from build123d import *

# Parameters (mm, degrees)
BOSS_EXTRUDE1_DEPTH = 6.35
FILLET1_R           = 3.81


with BuildPart() as part:
    # Sketch3 → Boss-Extrude1 (new body)
    with BuildSketch(Plane(origin=(809.076030053, 943.560396052, 1278.390464274), x_dir=(-1, 0, 0), z_dir=(0, 0.4075747752498649, -0.913171836282757))):
        with BuildLine():
            Line((137.874265639, -126.392405854), (-26.505638525, -18.937567822))
            Line((-26.505638525, -18.937567822), (-39.07644953, -10.720052017))
            ThreePointArc((-39.07644953, -10.720052017), (-20.260111199, -2.728624711), (0, 0))
            Line((0, 0), (320.198396744, 0))
            ThreePointArc((320.198396744, 0), (340.458416927, -2.728663039), (359.274618149, -10.720195518))
            Line((359.274618149, -10.720195518), (346.703910708, -18.937649247))
            Line((346.703910708, -18.937649247), (182.324265639, -126.392391447))
            ThreePointArc((182.324265639, -126.392391447), (160.099261742, -114.368537545), (137.874265639, -126.392405854))
        make_face()
    extrude(amount=BOSS_EXTRUDE1_DEPTH)

    # Fillet1
    fillet1_edges = [part.edges().sort_by_distance(p)[0] for p in [
        (671.201764414, 829.436460617, 1223.976787284),
        (848.152479583, 935.065196378, 1271.121920902),
        (449.801411904, 935.065065337, 1271.121862415),
        (626.751764414, 829.436473773, 1223.976793156),
    ]]
    fillet(fillet1_edges, radius=FILLET1_R)


solid = part.part
Read the model definition and answer for the solid it produces. Units are mm, in the model's axes. Round coordinates to 2 decimals unless told otherwise and drop trailing zeros. Write each loop counter-clockwise with the first axis right and the second up, starting at its lowest first coordinate (ties: lowest second). Pieces come first, ordered by that corner, then holes. Notation, with made-up numbers: M -36.75,43 L 2.25,43 A9 cw 2.25,52 Z; hole C -36,21.25 d8. An arc over 180 degrees is marked long. Use a Markdown table: item, result.
1) Flat-ended cylindrical pins translate along their axes: pin 1 (2 mm diameter, centred on x = 664, y = 861.5, fed in from -Z); pin 2 (5 mm diameter, centred on x = 625, y = 925, fed in from -Z); pin 3 (10 mm diameter, centred on x = 688.5, z = 1254.5, fed in from +Y). Find the tip coordinate at first contact, or state that the pin passes through.
Answers follow:
| item | result |
|---|---|
| pin 1 | stops at z = 1234.36 |
| pin 2 | stops at z = 1262.04 |
| pin 3 | stops at y = 916.82 |
2) The part is cut by section B-B (x = 598). Write down the section's boundary in (y, z).
Answers follow:
| item | result |
|---|---|
| outline | M 845.31,1234.54 L 847.89,1228.74 L 946.15,1272.59 L 943.56,1278.39 Z |
3) The part is cut by section A-A (y = 878). Write down the section's boundary in (x, z), plus the area to 3 significant figures.
Answers follow:
| item | result |
|---|---|
| outline | M 543.23,1249.13 L 547.57,1242.18 L 750.39,1242.18 L 754.72,1249.13 Z |
| area | 1,440 mm2 |
4) Straight lines are drawn through the part: line 1 along X through (y, z) = (932.5, 1267.5); line 2 along Z through (x, y) = (728, 891); line 3 along Y through (x, z) = (595.5, 1251). For each, find the intervals that lie inside material, in ascending order. Write a range as [from, to].
Answers follow:
| item | result |
|---|---|
| line 1 | x = [455.64, 842.31] |
| line 2 | z = [1247.98, 1254.93] |
| line 3 | y = [882.19, 897.77] |
